Check sheet for the drawn part. Datum: minimum x, y, z corner. Units: mm. A direction names the side the tool comes from. Round coordinates to 2 decimals unless told otherwise and drop trailing zeros. Loops run counter-clockwise (first coordinate to the right, second up) from the corner with the lowest first, then second, coordinate; pieces in that order, holes last. Notation, with made-up numbers: (-3, -25) -> (23, -25) arc R32 cw to (23, 5) -> close; hole circle Ø8 at (61.25, 52). An arc over 180 degrees is marked (long way). Return JSON: item names as keys, results as strings.
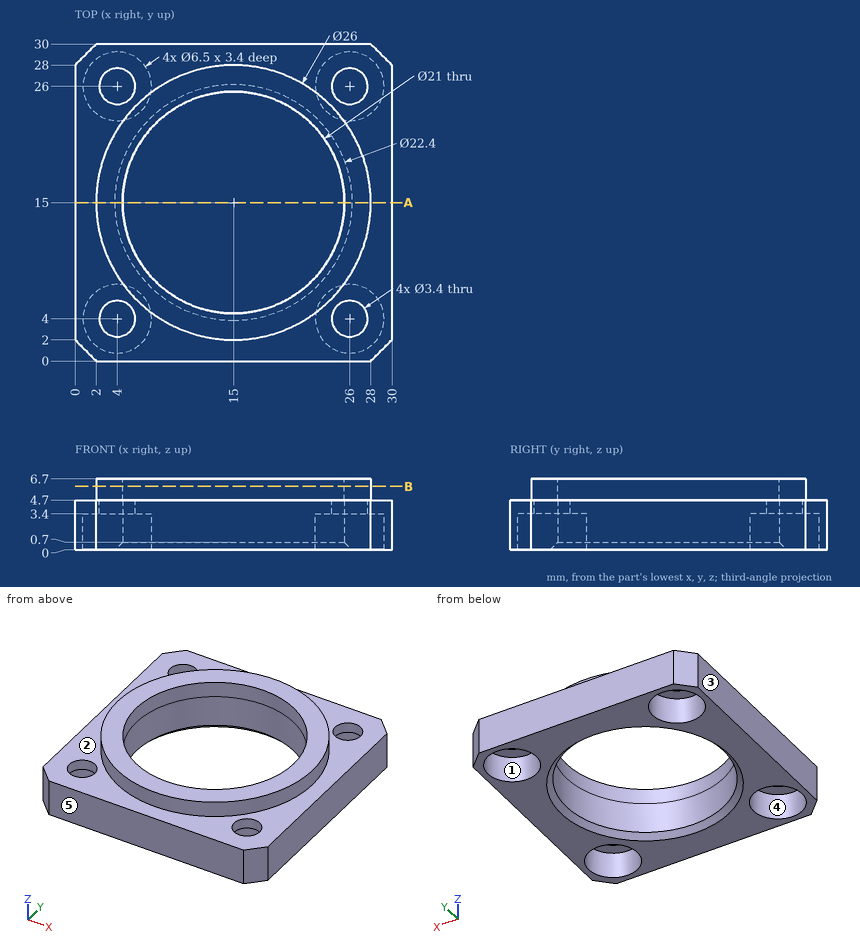
Q1. Draft check along X on the marked faces 1, 2 and 3. Enter one of: released by +X, released by -X, zero draft, split by the parting line, or undercut.
Results list:
{"face 1": "undercut", "face 2": "zero draft", "face 3": "released by -X"}
Q2. Tool access check on the marked faces 4 and 5. Record the directions out of +Z, -Z, +X, -X, +Y, -Y that give a thin tool (end or side, any length) a straight path to the whole face; none if there is none.
Results list:
{"face 4": "-Z", "face 5": "+Z, -Z, +X, -X, -Y"}
Q3. Material ranges on line 1 (Y direction, x = 26, z = 4); line 2 (Y direction, x = 26, z = 2.35), recorded low to high.
Results list:
{"line 1": "0 to 2.3, 5.7 to 24.3, 27.7 to 30", "line 2": "0 to 0.75, 7.25 to 22.75, 29.25 to 30"}
Q4. Section check A-A (y = 15). Record the boundary of the cut face in (x, z).
Results list:
{"outline": "(0, 0) -> (3.8, 0) -> (4.5, 0.7) -> (4.5, 6.7) -> (2, 6.7) -> (2, 4.7) -> (0, 4.7) -> close; (25.5, 0.7) -> (26.2, 0) -> (30, 0) -> (30, 4.7) -> (28, 4.7) -> (28, 6.7) -> (25.5, 6.7) -> close"}
Q5. Go/stop test with flat-tipped pins: pin 1 (6 mm diameter, centred on x = 4, y = 26, fed in from -Z); pin 2 (6 mm diameter, centred on x = 24.5, y = 14, fed in from -Z); pin 3 (17 mm diameter, centred on x = 15, y = 15, fed in from +Z). Record where each tip stops, or that it passes through.
Results list:
{"pin 1": "z = 3.4", "pin 2": "z = 0", "pin 3": "through"}
Q6. Section check B-B (z = 6). Record the boundary of the cut face in (x, y).
Results list:
{"outline": "circle Ø26 at (15, 15); hole circle Ø21 at (15, 15)"}
